Autodesk Inventor part; units mm, degrees
ref_plane "YZ Plane" through (0, 0, 0) normal (1, 0, 0) x (0, 1, 0)
ref_plane "XZ Plane" through (0, 0, 0) normal (0, 1, 0) x (-1, 0, 0)
ref_plane "XY Plane" through (0, 0, 0) normal (0, 0, 1) x (1, 0, 0)
sketch "Sketch1" plane through (0, 0, 0) normal (0, 1, 0) x (-1, 0, 0)
  circle A0 centre (0, 0) radius 4.375
  circle A1 centre (1.8, 1.5) radius 1.25
  circle A2 centre (1.5, -1.5) radius 1.25
  circle A3 centre (-1.8, 1.5) radius 1.25
  circle A4 centre (-1.5, -1.5) radius 1.25
  line L0 (1.4885, 4.7346) -> (0.1984, 4.7346)
  line L1 (-1.5115, 4.1056) -> (-1.5115, 3.4074)
  line L2 (-1.5115, 3.4074) -> (1.4885, 3.4074)
  line L3 (1.4885, 3.4074) -> (1.4885, 4.7346)
  line L4 (1.4885, 4.7346) -> (-1.5115, 3.4074) construction
  line L5 (0.1984, 4.7346) -> (1.4885, 3.4074) construction
  line L6 (2.1288, -3.5803) -> (-2.1422, -3.5803)
  line L7 (-2.1422, -3.5803) -> (-2.1422, -3.8146)
  line L8 (-2.1708, -5.1794) -> (2.1288, -5.1794)
  line L9 (2.1288, -5.1794) -> (2.1288, -3.5803)
  line L10 (4.2592, 1) -> (3.375, 1)
  line L11 (3.375, 1) -> (3.375, -1)
  line L12 (3.375, -1) -> (5.375, -1)
  line L13 (5.375, -1) -> (5.375, 1)
  line L14 (5.375, 1) -> (3.375, -1) construction
  line L15 (3.375, 1) -> (5.375, -1) construction
  line L16 (-3.375, 1) -> (-4.2592, 1)
  line L17 (-5.375, 1) -> (-5.375, -1)
  line L18 (-5.375, -1) -> (-3.375, -1)
  line L19 (-3.375, -1) -> (-3.375, 1)
  line L20 (-3.375, 1) -> (-5.375, -1) construction
  line L21 (-5.375, 1) -> (-3.375, -1) construction
  point P0 (0.5864, 4.3355)
  point P1 (0.2908, -4.3653)
  point P2 (1.4885, 4.114)
  point P3 (2.1288, -3.8221)
  point P4 (4.375, 0)
  point P5 (-4.375, 0)
  point P6 (-4.2592, -1)
  point P7 (4.2592, -1)
  dimension "d0" = 8.75
  dimension "d1" = 2.5
  dimension "d_1" = 2.5
  dimension "d3" = 2.5
  dimension "d4" = 2.5
  dimension "d5" = 1.5
  dimension "d6" = 1.5
  dimension "d7" = 1.5
  dimension "d8" = 1.5
  dimension "d9" = 1.8
  dimension "d10" = 1.8
  dimension "d11" = 1.5
  dimension "d12" = 1.5
  dimension "d13" = 3
  dimension "d19" = 2
  dimension "d20" = 2
  dimension "d21" = 2
  dimension "d22" = 2
extrude "Extrusion1" add sketch "Sketch1" along normal blind 6 contours L10 L11 L12 A0 L9 L6 L7 L18 L19 L16 L1 L2 L3
sketch "Sketch2" plane through (0, 0, 0) normal (0, -1, 0) x (1, 0, 0)
  circle A0 centre (1.5, -1.5) radius 1.25
  circle A1 centre (1.8, 1.5) radius 1.25
  circle A2 centre (-1.5, -1.5) radius 1.25
  circle A3 centre (-1.8, 1.5) radius 1.25
  line L0 (1.5115, 3.4074) -> (1.5115, 4.1056)
  line L1 (-1.4885, 3.4074) -> (1.5115, 3.4074)
  line L2 (-1.4885, 4.114) -> (-1.4885, 3.4074)
  arc A4 (-1.4885, 4.114) -> (-4.2592, 1) centre (0, 0) ccw
  line L3 (-3.375, 1) -> (-4.2592, 1)
  line L4 (-3.375, -1) -> (-3.375, 1)
  line L5 (-4.2592, -1) -> (-3.375, -1)
  arc A5 (-4.2592, -1) -> (-2.1288, -3.8221) centre (0, 0) ccw
  line L6 (-2.1288, -3.5803) -> (-2.1288, -3.8221)
  line L7 (2.1422, -3.5803) -> (-2.1288, -3.5803)
  line L8 (2.1422, -3.8146) -> (2.1422, -3.5803)
  arc A6 (2.1422, -3.8146) -> (4.2592, -1) centre (0, 0) ccw
  line L9 (3.375, -1) -> (4.2592, -1)
  line L10 (3.375, 1) -> (3.375, -1)
  line L11 (4.2592, 1) -> (3.375, 1)
  arc A7 (4.2592, 1) -> (1.5115, 4.1056) centre (0, 0) ccw
  circle A8 centre (0, 0) radius 5.9296
equation "\"d1\" = d_1"
equation "\"d3\" = d_1"
equation "\"d4\" = d_1"
properties part number "00_Kycon_4pin_mail"
Input: part model. Units: mm. Frame: model coordinates. A direction names the side the tool comes from. Give positions to 0.01 mm unless a question says otherwise; leave off trailing zeros. Write each loop counter-clockwise with the first axis right and the second up, starting at its lowest first coordinate (ties: lowest second). Pieces come first, ordered by that corner, then holes. Notation, with made-up numbers: (24.25, -37) -> (38.25, -37) arc R18 cw to (38.25, -4) -> close; hole circle Ø3 at (-8.5, 57). An arc over 180 degrees is marked (long way). Use one line per item in the form item = value. Start each with the question number.
1) Section query C-C on z = -0.5. Return the cut outline in (x, y) (3 decimals), then the cut area to 3 significant figures.
2) Set-up query: faces 1 (the flat face through (4, 3, -1)), 2 (the flat face through (0, 3, 3.407)), 3 (the flat face through (-4, 3, 1)), 4 (the flat face through (0, 3, -3.58)). Return all of +Z, -Z, +X, -X, +Y, -Y with unobstructed straight access to the full face (end or side cutting, diameter ignored); none if empty.
3) Ray query, probe 1 along Z at (x, y) = (2, 4.6); probe 2 along Z at (x, y) = (-1, 1.5); probe 3 along X at (y, z) = (4.1, -2.5). Return the intervals inside material, ascending. Write a range as from..to.
4) Draft query along Z for faces 5 (the cylindrical face through (3.48, 2.96, -2.65)), 6 (the flat face through (4, 3, 1)), 7 (the cylindrical face through (-3.25, 2.96, 2.93)), 8 (the cylindrical face through (-2.955, 2.958, 1.979)). Return one class per face: pulls with the +Z half, pulls with the -Z half, needs draft (parallel to the pull), parting line crosses it, or undercut.
5) Section query A-A on z = 0.75. Return the cut outline in (x, y) (3 decimals), then the cut area to 3 significant figures.
6) Section query B-B on y = 1.8. Count the separate pieces of the cut face and the enclosed holes in it, then the cut area to 3 significant figures.
7) Pin query (flat end, axial travel): pin 1 (0.6 mm diameter, centred on y = 1.5, z = 0, fed in from +X) (3 decimals); pin 2 (3 mm diameter, centred on x = 0.5, y = 4, fed in from -Z); pin 3 (0.8 mm diameter, centred on y = 2.5, z = 4, fed in from -X). Return the tip coordinate at first contact, or that it passes through.
Outcome:
q1.outline = (-3.375, 0) -> (-2.25, 0) -> (-2.25, 6) -> (-3.375, 6) -> close; (-0.75, 0) -> (0.75, 0) -> (0.75, 6) -> (-0.75, 6) -> close; (2.25, 0) -> (3.375, 0) -> (3.375, 6) -> (2.25, 6) -> close
q1.area = 22.5 mm^2
q2.face_1 = +X, +Y, -Y
q2.face_2 = +Z, +Y, -Y
q2.face_3 = -X, +Y, -Y
q2.face_4 = -Z, +Y, -Y
q3.probe_1 = -3.58..-2.65, -0.35..0.27, 2.73..3.89
q3.probe_2 = -3.58..-2.65, -0.35..0.54, 2.46..3.41
q3.probe_3 = -3.59..-2.25, -0.75..0.75, 2.25..3.59
q4.face_5 = pulls with the -Z half
q4.face_6 = undercut
q4.face_7 = pulls with the +Z half
q4.face_8 = undercut
q5.outline = (-3.375, 0) -> (-2.8, 0) -> (-2.8, 6) -> (-3.375, 6) -> close; (-0.8, 0) -> (0.8, 0) -> (0.8, 6) -> (-0.8, 6) -> close; (2.8, 0) -> (3.375, 0) -> (3.375, 6) -> (2.8, 6) -> close
q5.area = 16.5 mm^2
q6.separate_pieces = 1
q6.enclosed_holes = 4
q6.area = 31.4 mm^2
q7.pin_1 = 3.375
q7.pin_2 = -3.58
q7.pin_3 = -2.49
